from build123d import *

# Parameters (mm, degrees)
F1_DEPTH = 6.35
F3_DEPTH = 38.1


with BuildPart() as f1:
    # F0 (on Right) → F1 (new body, symmetric)
    with BuildSketch(Plane.YZ):
        with BuildLine():
            Line((24.33887, 4.155473), (-21.92162, 4.155473))
            ThreePointArc((-21.92162, 4.155473), (-24.056937, 3.330164), (-25.082145, 1.283298))
            Line((-25.082145, 1.283298), (-25.082145, -8.879172))
            ThreePointArc((-25.082145, -8.879172), (-24.489592, -10.726222), (-22.93311, -11.883839))
            Line((-22.93311, -11.883839), (-9.41385, -16.500088))
            ThreePointArc((-9.41385, -16.500088), (-7.628749, -16.835147), (-5.821818, -16.65116))
            Line((-5.821818, -16.65116), (22.703972, -9.519713))
            ThreePointArc((22.703972, -9.519713), (26.168975, -7.267175), (27.51387, -3.359308))
            Line((27.51387, -3.359308), (27.51387, 0.980473))
            ThreePointArc((27.51387, 0.980473), (26.583934, 3.225537), (24.33887, 4.155473))
        make_face()
    extrude(amount=F1_DEPTH, both=True)

    # F2 (on Front) → F3 (cut, symmetric)
    with BuildSketch(Plane.XZ):
        Polygon((-6.35, -6.35), (0, 0), (0, 6.35), (-12.7, 6.35), (-12.7, -6.35), align=None)
    extrude(amount=F3_DEPTH, both=True, mode=Mode.SUBTRACT)


solid = f1.part
The listing builds one solid part. Answer for the finished solid, in the listing's coordinates (mm). Give positions to 0.01 mm unless a question says otherwise; leave off trailing zeros. Loops run counter-clockwise (first coordinate to the right, second up) from the corner with the lowest first, then second, coordinate; pieces in that order, holes last.
Item 1: Determine the mould class of faces 1 (the cylindrical face through (3.219, -24.033, 3.352)), 2 (the flat face through (6.35, 1, -4)), 3 (the flat face through (0, 1, 2)) for opening direction X: +X half, -X half, draft (parallel to the pull), parting line (faces both ways), or undercut.
Derived:
face 1: draft
face 2: +X half
face 3: -X half
Item 2: A cutting plane is placed at B-B (x = 4.75). Give the vertices of the cut face in (y, z) (3 decimals), then the cut area to 3 significant figures.
Derived:
outline: (-25.082, -8.879) arc R3.175 ccw to (-22.933, -11.884) - (-9.414, -16.5) arc R6.35 ccw to (-5.822, -16.651) - (22.704, -9.52) arc R6.35 ccw to (27.514, -3.359) - (27.514, 0.98) arc R3.175 ccw to (24.339, 4.155) - (-21.922, 4.155) arc R3.175 ccw to (-25.082, 1.283) - close
area: 902 mm2
Item 3: A cutting plane is placed at D-D (z = -14). Give the vertices of the cut face in (x, y).
Derived:
outline: (-6.35, -16.74) - (6.35, -16.74) - (6.35, 4.78) - (-6.35, 4.78) - close
Item 4: This flat-tipped pin is pushed along its axis until it touches: pin 1 Ø1.2 at (y, z) = (0, 2) entering from -X. Where does it stop, or does it pass through?
Derived:
pin 1: stops at x = 0
Item 5: Find the intervals of material crossed by line 1 along Z through (x, y) = (4, -7); line 2 along X through (y, z) = (-13, -3.5); line 3 along Y through (x, z) = (0.75, -7.5), in increasing order.
Derived:
line 1: z = -16.83 to 4.16
line 2: x = -3.5 to 6.35
line 3: y = -25.08 to 25.98
Item 6: A cutting plane is placed at A-A (x = -1.5). Give the vertices of the cut face in (y, z) (3 decimals), then the cut area to 3 significant figures.
Derived:
outline: (-25.082, -8.879) arc R3.175 ccw to (-22.933, -11.884) - (-9.414, -16.5) arc R6.35 ccw to (-5.822, -16.651) - (22.704, -9.52) arc R6.35 ccw to (27.514, -3.359) - (27.514, -1.5) - (-25.082, -1.5) - close
area: 608 mm2
Item 7: A cutting plane is placed at C-C (y = -19.5). Give the vertices of the cut face in (x, z).
Derived:
outline: (-6.35, -13.06) - (6.35, -13.06) - (6.35, 4.16) - (0, 4.16) - (0, 0) - (-6.35, -6.35) - close
